The model under review builds one solid part; all positions refer to its coordinate system, in mm. Round coordinates to 2 decimals unless told otherwise and drop trailing zeros. Order: outer loops, then holes, each group sorted by start corner. A loop starts at its lowest first (then second) coordinate and runs counter-clockwise, first axis right, second up. Notation, with made-up numbers: (-22.75, 28) -> (9.25, 28) arc R12 cw to (9.25, 46) -> close; hole circle Ø5 at (25, 52). An arc over 180 degrees is marked (long way). Return JSON: item names as keys, results as strings. Group by question number.
from build123d import *

# Parameters (mm, degrees)
ODGI_CIE_BAZOWE1_DEPTH     = 400
WYTNIJ_WYCI_GNI_CIE1_REACH = 404.676
OTWORY_POD_NITY_R          = 2
WYTNIJ_WYCI_GNI_CIE2_DEPTH = 403.618628481


# Sheet-metal steps are written as plain solids
with BuildPart() as part:
    # Szkic1 → Odgięcie bazowe1 (new body)
    with BuildSketch(Plane(origin=(0, 0, 0), x_dir=(1, 0, 0), z_dir=(0, 1, 0))):
        with BuildLine():
            ThreePointArc((4.952776999, 1.1), (-2.536730179, 23.121689892), (0, 0))
            Line((0, 0), (40, 0))
            Line((40, 0), (40, 1))
            Line((40, 1), (0, 1))
            ThreePointArc((0, 1), (-2.319915634, 22.145477081), (4.529462725, 2.005982906))
            Line((4.529462725, 2.005982906), (4.952776999, 1.1))
        make_face()
    extrude(amount=-ODGI_CIE_BAZOWE1_DEPTH)

    # Szkic6 → Wytnij-wyciągnięcie1 (cut, up to next)
    with BuildSketch(Plane.XY, mode=Mode.PRIVATE) as wytnij_wyci_gni_cie1_sk1:
        with BuildLine():
            Line((0, 0), (0, -20))
            Line((0, -20), (35, -20))
            ThreePointArc((35, -20), (38.535533906, -21.464466094), (40, -25))
            Line((40, -25), (40, -20))
            Line((40, -20), (40, 0))
            Line((40, 0), (0, 0))
        make_face()
    wytnij_wyci_gni_cie1_tool1 = extrude(wytnij_wyci_gni_cie1_sk1.sketch, amount=-WYTNIJ_WYCI_GNI_CIE1_REACH, mode=Mode.PRIVATE) & part.part
    add(wytnij_wyci_gni_cie1_tool1.solids().sort_by_distance((20.125793, -10.074056, 0))[0], mode=Mode.SUBTRACT)

    # otwory pod nity → Wytnij-wyciągnięcie2 (cut, through all)
    with BuildSketch(Plane(origin=(0, 0, -1), x_dir=(-1, 0, 0), z_dir=(0, 0, -1))):
        with Locations((-35, -25)):
            Circle(OTWORY_POD_NITY_R)
        with Locations(Location((-16.7, -25, 0), (0, 0, 180))):
            Circle(OTWORY_POD_NITY_R)
        with Locations((-16.7, -395)):
            Circle(OTWORY_POD_NITY_R)
        with Locations(Location((-35, -395, 0), (0, 0, 180))):
            Circle(OTWORY_POD_NITY_R)
        with BuildLine():
            Line((-35, -400), (-40, -400))
            Line((-40, -400), (-40, -395))
            ThreePointArc((-40, -395), (-38.535533906, -398.535533906), (-35, -400))
        make_face()
    extrude(amount=-WYTNIJ_WYCI_GNI_CIE2_DEPTH, mode=Mode.SUBTRACT)


solid = part.part
Item 1: The part is to be moulded in two halves that separate along Z. For faces 1 (the face through (20, -207, -1)), 2 (the face through (20, -207, 0)), 3 (the face through (10, -400, -7)), say which applies: +Z half, -Z half, draft (parallel to the pull), parting line (faces both ways), or undercut.
Item 2: Wall thickness on line 1 along Y through (x, z) = (35, -0.3); line 2 along Z through (x, y) = (1, -186.5); line 3 along X through (y, z) = (-351, -12.5): over which ranges is each line inside the solid? List them lowest first.
Item 3: Insertion check: pin 1 Ø5 at (x, y) = (27.5, -308.5) entering from +Z; pin 2 Ø1.1 at (y, z) = (-11, -0.5) entering from +X; pin 3 Ø20 at (x, y) = (23.5, -296.5) entering from -Z; pin 4 Ø0.5 at (x, z) = (11.5, -0.5) entering from +Y. Each pin has a flat end and moves straight along its axis. Give the tip position at first contact, or say it passes through.
Item 4: Consider section C-C on y = -157.5. State the section outline as (x, z) points.
Item 5: Consider section B-B on x = -4. State the section outline as (y, z) points (3 decimals), plus the area to 3 significant figures.
Item 6: Consider section A-A on z = -11.7. State the section outline as (x, y) points.
Values:
{
 "1": {"face 1": "undercut", "face 2": "+Z half", "face 3": "draft"},
 "2": {"line 1": "-400 to -397, -393 to -27, -23 to -20", "line 2": "-23.36 to -22.35, -1 to 0", "line 3": "-11.67 to -10.67, 10.67 to 11.67"},
 "3": {"pin 1": "z = 0", "pin 2": "x = 0", "pin 3": "z = -1", "pin 4": "y = -20"},
 "4": {"outline": "(0, -1) -> (40, -1) -> (40, 0) -> (0, 0) arc R11.7 ccw (long way) to (4.95, -1.1) -> (4.53, -2.01) arc R10.7 cw (long way) to start"},
 "5": {"outline": "(-400, -22.695) -> (0, -22.695) -> (0, -21.624) -> (-400, -21.624) -> close; (-400, -1.776) -> (0, -1.776) -> (0, -0.705) -> (-400, -0.705) -> close", "area": "857 mm^2"},
 "6": {"outline": "(-11.7, -400) -> (-10.7, -400) -> (-10.7, 0) -> (-11.7, 0) -> close; (10.7, -400) -> (11.7, -400) -> (11.7, 0) -> (10.7, 0) -> close"}
}
